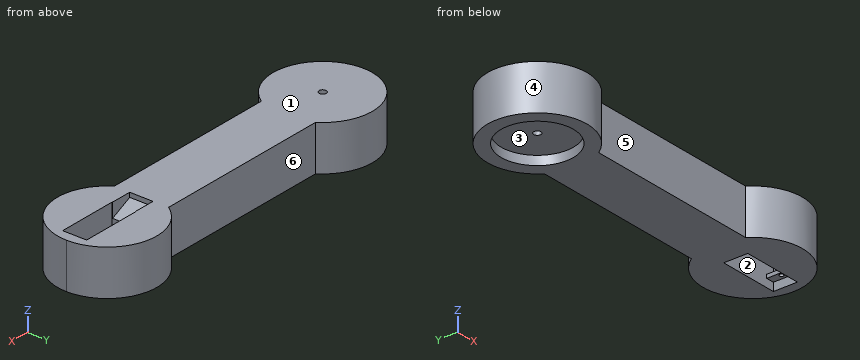
from build123d import *

# Parameters (mm, degrees)
BOSS_EXTRUDE1_DEPTH = 25
SKETCH16_W          = 33.4
SKETCH16_H          = 13.3
CUT_EXTRUDE10_DEPTH = 4.5
SKETCH19_R          = 20
CUT_EXTRUDE14_DEPTH = 5
SKETCH17_W          = 24.4
SKETCH17_H          = 13.3
CUT_EXTRUDE11_DEPTH = 177.45821035
CUT_EXTRUDE13_DEPTH = 6.45
SKETCH20_W          = 33.4
SKETCH20_H          = 13.3
CUT_EXTRUDE15_DEPTH = 176.655202029
SKETCH21_R          = 1.1
CUT_EXTRUDE16_DEPTH = 177.45821035
SKETCH22_R          = 2
CUT_EXTRUDE17_DEPTH = 20


with BuildPart() as part:
    # Sketch1 → Boss-Extrude1 (new body)
    with BuildSketch(Plane.XY):
        with BuildLine():
            ThreePointArc((172.5, 0), (152.823244805, 26.363741023), (121.951138857, 15))
            Line((121.951138857, 15), (145, 15))
            Line((145, 15), (145, -15))
            Line((145, -15), (121.951138857, -15))
            ThreePointArc((121.951138857, -15), (152.823244805, -26.363741023), (172.5, 0))
        make_face()
        with BuildLine():
            Line((145, 15), (121.951138857, 15))
            ThreePointArc((121.951138857, 15), (117.5, 0), (121.951138857, -15))
            Line((121.951138857, -15), (145, -15))
            Line((145, -15), (145, 15))
        make_face()
        with BuildLine():
            Line((121.951138857, 15), (23.048861143, 15))
            ThreePointArc((23.048861143, 15), (26.363741023, 7.823244805), (27.5, 0))
            ThreePointArc((27.5, 0), (26.363741023, -7.823244805), (23.048861143, -15))
            Line((23.048861143, -15), (121.951138857, -15))
            ThreePointArc((121.951138857, -15), (117.5, 0), (121.951138857, 15))
        make_face()
        with BuildLine():
            ThreePointArc((13.228756555, -15), (-20, 0), (13.228756555, 15))
            Line((13.228756555, 15), (23.048861143, 15))
            ThreePointArc((23.048861143, 15), (-27.5, 0), (23.048861143, -15))
            Line((23.048861143, -15), (13.228756555, -15))
        make_face()
        with BuildLine():
            Line((23.048861143, 15), (13.228756555, 15))
            ThreePointArc((13.228756555, 15), (18.228756555, 8.228756555), (20, 0))
            ThreePointArc((20, 0), (18.228756555, -8.228756555), (13.228756555, -15))
            Line((13.228756555, -15), (23.048861143, -15))
            ThreePointArc((23.048861143, -15), (26.363741023, -7.823244805), (27.5, 0))
            ThreePointArc((27.5, 0), (26.363741023, 7.823244805), (23.048861143, 15))
        make_face()
        with BuildLine():
            Line((0, -15), (0, 15))
            Line((0, 15), (13.228756555, 15))
            ThreePointArc((13.228756555, 15), (-20, 0), (13.228756555, -15))
            Line((13.228756555, -15), (0, -15))
        make_face()
        with BuildLine():
            Line((13.228756555, 15), (0, 15))
            Line((0, 15), (0, -15))
            Line((0, -15), (13.228756555, -15))
            ThreePointArc((13.228756555, -15), (18.228756555, -8.228756555), (20, 0))
            ThreePointArc((20, 0), (18.228756555, 8.228756555), (13.228756555, 15))
        make_face()
    extrude(amount=BOSS_EXTRUDE1_DEPTH)

    # Sketch16 → Cut-Extrude10 (cut)
    with BuildSketch(Plane(origin=(0, 0, 0), x_dir=(-1, 0, 0), z_dir=(0, 0, -1))):
        with Locations((-150.21934279, 0)):
            Rectangle(SKETCH16_W, SKETCH16_H)
    extrude(amount=-CUT_EXTRUDE10_DEPTH, mode=Mode.SUBTRACT)

    # Sketch19 → Cut-Extrude14 (cut)
    with BuildSketch(Plane(origin=(0, 0, 0), x_dir=(-1, 0, 0), z_dir=(0, 0, -1))):
        Circle(SKETCH19_R)
    extrude(amount=-CUT_EXTRUDE14_DEPTH, mode=Mode.SUBTRACT)

    # Sketch17 → Cut-Extrude11 (cut, through all)
    with BuildSketch(Plane(origin=(0, 0, 0), x_dir=(-1, 0, 0), z_dir=(0, 0, -1))):
        with Locations((-150.21934279, 0)):
            Rectangle(SKETCH17_W, SKETCH17_H)
    extrude(amount=-CUT_EXTRUDE11_DEPTH, mode=Mode.SUBTRACT)

    # Sketch18 → Cut-Extrude13 (cut, symmetric)
    with BuildSketch(Plane(origin=(0, 0, 0), x_dir=(-1, 0, 0), z_dir=(0, -1, 0))):
        Polygon((-138.01934279, -15), (-138.01934279, -25), (-122.01934279, -25), (-122.01934279, -22.5), align=None)
    extrude(amount=CUT_EXTRUDE13_DEPTH, both=True, mode=Mode.SUBTRACT)

    # Sketch20 → Cut-Extrude15 (cut, through all)
    with BuildSketch(Plane(origin=(0, 0, 6.5), x_dir=(-1, 0, 0), z_dir=(0, 0, -1))):
        with Locations((-150.21934279, 0)):
            Rectangle(SKETCH20_W, SKETCH20_H)
    extrude(amount=-CUT_EXTRUDE15_DEPTH, mode=Mode.SUBTRACT)

    # Sketch21 → Cut-Extrude16 (cut, through all)
    with BuildSketch(Plane(origin=(0, 0, 0), x_dir=(-1, 0, 0), z_dir=(0, 0, -1))):
        with Locations((-164.249999957, 0)):
            Circle(SKETCH21_R)
        with Locations((-136.249999957, 0)):
            Circle(SKETCH21_R)
    extrude(amount=-CUT_EXTRUDE16_DEPTH, mode=Mode.SUBTRACT)

    # Sketch22 → Cut-Extrude17 (cut)
    with BuildSketch(Plane.XY.offset(25)):
        Circle(SKETCH22_R)
    extrude(amount=-CUT_EXTRUDE17_DEPTH, mode=Mode.SUBTRACT)


solid = part.part
Build history of the part. All positions in model axes, mm. Face numbers are marked on the shaded views. A direction names the side the tool comes from. Coordinates: 2 decimals unless noted, no trailing zeros. Order: outer loops, then holes, each group sorted by start corner. A loop starts at its lowest first (then second) coordinate and runs counter-clockwise, first axis right, second up. Notation, with made-up numbers: M -20,36 L 28,36 A23 ccw 28,54 Z; hole C 88,19.25 d9. An arc over 180 degrees is marked long. One line per question, with ' | ' between items. Start each with the question number.
Q1. Saw through at B-B (z = 2). List the corners of the cut face in (x, y).
Q2. Saw through at D-D (x = 88). List the corners of the cut face in (y, z), then the cut area to 3 significant figures.
Q3. 3-axis set-ups, long thin cutter, end or side, ignore diameter. For the marked faces 3, 4, 5 and 6: which of +Z, -Z, +X, -X, +Y, -Y reach the whole face in a straight line?
Q4. Flat gauge pins, fed straight in: pin 1 Ø12.5 at (x, z) = (51.5, 8) entering from +Y; pin 2 Ø5 at (x, y) = (3, -14.5) entering from -Z; pin 3 Ø8.5 at (x, z) = (126.5, 22) entering from -Y. Where does each tip first touch, or does it go through?
Q5. Probe L1, parallel to X at y = 0.5, z = 1.5; L2, parallel to X at y = -1, z = 7.25; L3, parallel to Y at x = 0, z = 11.75. List the from-to ranges inside material, lowest first. Write a range as from..to.
Q6. Saw through at C-C (z = 12). List the corners of the cut face in (x, y), then the cut area to 3 significant figures.
Q7. Two-plate mould, pull along X, no slides. Class the marked faces 1 and 2: +X half, -X half, draft (parallel to the pull), parting line (faces both ways), or undercut.
Q8. Saw through at A-A (x = 0). List the corners of the cut face in (y, z), then the cut area to 4 significant figures.
Check values:
1) outline: M 23.05,-15 L 121.95,-15 A27.5 ccw long 121.95,15 L 23.05,15 A27.5 ccw long Z; hole C 0,0 d40; hole M 133.52,-6.65 L 166.92,-6.65 L 166.92,6.65 L 133.52,6.65 Z
2) outline: M -15,0 L 15,0 L 15,25 L -15,25 Z | area: 750 mm2
3) face 3: -Z | face 4: +Z, -Z | face 5: +Z, -Z, -Y | face 6: +Z, -Z, +Y
4) pin 1: stops at y = 15 | pin 2: stops at z = 5 | pin 3: stops at y = -23.52
5) L1: x = -27.5..-19.99, 19.99..133.52, 166.92..172.5 | L2: x = -27.48..-1.73, 1.73..133.52, 166.92..172.48 | L3: y = -27.5..-2, 2..27.5
6) outline: M 23.05,-15 L 121.95,-15 A27.5 ccw long 121.95,15 L 23.05,15 A27.5 ccw long Z; hole C 0,0 d4; hole M 133.52,-6.65 L 166.92,-6.65 L 166.92,6.65 L 133.52,6.65 Z | area: 7,080 mm2
7) face 1: draft | face 2: undercut
8) outline: M -27.5,0 L -20,0 L -20,5 L -2,5 L -2,25 L -27.5,25 Z; M 2,5 L 20,5 L 20,0 L 27.5,0 L 27.5,25 L 2,25 Z | area: 1,095 mm2
